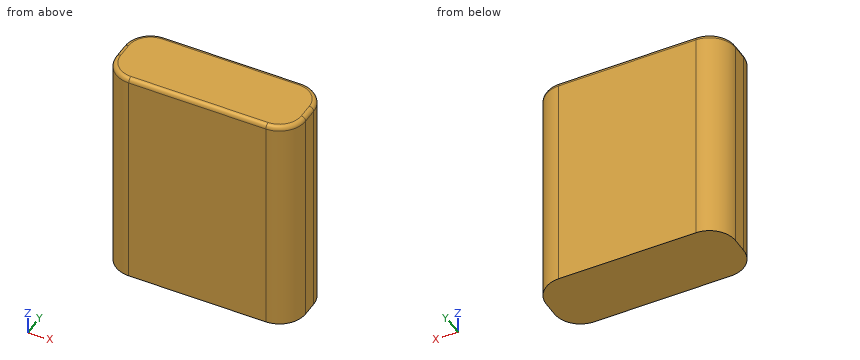
```python
from build123d import *

# Parameters (mm, degrees)
BOSS_EXTRUDE1_DEPTH = 52
FILLET1_R           = 1


with BuildPart() as part:
    # Sketch2 → Boss-Extrude1 (new body)
    with BuildSketch(Plane.XY):
        with BuildLine():
            Line((-15.75, -7.75), (15.75, -7.75))
            ThreePointArc((15.75, -7.75), (19.992640687, -5.992640687), (21.75, -1.75))
            Line((21.75, -1.75), (21.75, 1.75))
            ThreePointArc((21.75, 1.75), (19.992640687, 5.992640687), (15.75, 7.75))
            Line((15.75, 7.75), (-15.75, 7.75))
            ThreePointArc((-15.75, 7.75), (-19.992640687, 5.992640687), (-21.75, 1.75))
            Line((-21.75, 1.75), (-21.75, -1.75))
            ThreePointArc((-21.75, -1.75), (-19.992640687, -5.992640687), (-15.75, -7.75))
        make_face()
    extrude(amount=BOSS_EXTRUDE1_DEPTH)

    # Fillet1
    fillet1_edges = [part.edges().sort_by_distance(p)[0] for p in [
        (-19.992640687, 5.992640687, 52),
        (-21.75, 0, 52),
        (-19.992640687, -5.992640687, 52),
        (0, -7.75, 52),
        (19.992640687, -5.992640687, 52),
        (21.75, 0, 52),
        (19.992640687, 5.992640687, 52),
        (0, 7.75, 52),
    ]]
    fillet(fillet1_edges, radius=FILLET1_R)


solid = part.part
```
Model file for the job. Use its own axes, mm. Coordinates: 2 decimals unless noted, no trailing zeros. Order: outer loops, then holes, each group sorted by start corner. A loop starts at its lowest first (then second) coordinate and runs counter-clockwise, first axis right, second up. Notation, with made-up numbers: (-33.5, 37.5) -> (-13.5, 37.5) arc R7 ccw to (-13.5, 46.5) -> close; hole circle Ø3 at (-22.75, -4.75). An arc over 180 degrees is marked (long way). Answer as a JSON object with one key per item and string values. Group by question number.
1) Drill centre lines: L1, parallel to X at y = -2, z = 2; L2, parallel to X at y = 3.5, z = 30; L3, parallel to Y at x = 16, z = 8. Where is each one in solid material? Low to high.
2) Cut at A-A, the plane z = 47. Write the cut outline in (x, y), then the cut area to 3 significant figures.
3) Flat gauge pins, fed straight in: pin 1 (2 mm diameter, centred on y = -3, z = 42.5, fed in from -X); pin 2 (4 mm diameter, centred on y = -5, z = 46, fed in from -X); pin 3 (1 mm diameter, centred on y = -6, z = 24.5, fed in from +X). Where does each tip first touch, or does it go through?
Check values:
{
 "1": {"L1": "x = -21.74 to 21.74", "L2": "x = -21.49 to 21.49", "L3": "y = -7.74 to 7.74"},
 "2": {"outline": "(-21.75, -1.75) arc R6 ccw to (-15.75, -7.75) -> (15.75, -7.75) arc R6 ccw to (21.75, -1.75) -> (21.75, 1.75) arc R6 ccw to (15.75, 7.75) -> (-15.75, 7.75) arc R6 ccw to (-21.75, 1.75) -> close", "area": "643 mm²"},
 "3": {"pin 1": "stops at x = -21.74", "pin 2": "stops at x = -21.62", "pin 3": "stops at x = 20.43"}
}
